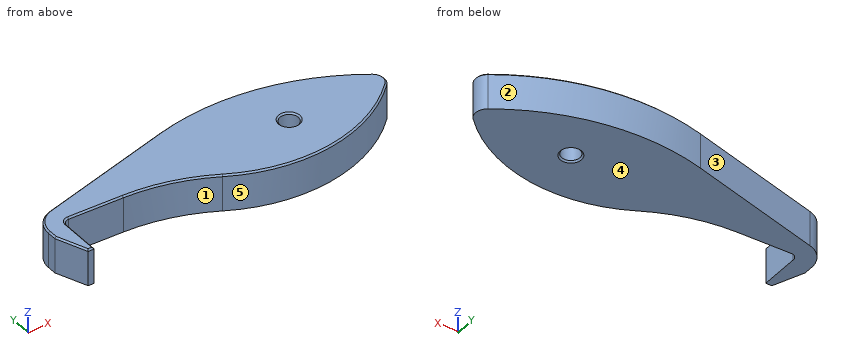
Autodesk Inventor part; units mm, degrees
ref_plane "YZ Plane" through (0, 0, 0) normal (1, 0, 0) x (0, 1, 0)
ref_plane "XZ Plane" through (0, 0, 0) normal (0, 1, 0) x (-1, 0, 0)
ref_plane "XY Plane" through (0, 0, 0) normal (0, 0, 1) x (1, 0, 0)
sketch "Náčrt1" plane through (0, 0, 0) normal (0, 0, 1) x (1, 0, 0)
  line L0 (-106.433, 0) -> (55.3696, 0)
  line L1 (0, -81.7425) -> (0, 52.651)
  circle A0 centre (0, 0) radius 3
  arc A1 (30.8349, -1.8219) -> (30.2938, 4.277) centre (28, 1) ccw
  arc A2 (-76.0338, 3.7372) -> (-82, -4) centre (-74, -4) ccw
  arc A3 (-73.9347, -2.0011) -> (-75.9978, -4.0942) centre (-74, -4) ccw
  line L2 (-75.9978, -3.9058) -> (-75.9978, -16.9058)
  line L3 (-75.9978, -16.9058) -> (-77.9978, -16.9058)
  line L4 (-77.9978, -16.9058) -> (-82, -7)
  line L5 (-82, -4) -> (-82, -7)
  arc A4 (30.2938, 4.277) -> (-31.7818, 15.3695) centre (-12.7146, -57.1663) ccw
  arc A5 (-29.0159, -10.1823) -> (30.8349, -1.8219) centre (-4.6017, 33.4519) ccw
  arc A6 (-29.0159, -10.1823) -> (-56.3536, -2.5755) centre (-58.3128, -62.5435) ccw
  line L6 (-76.0338, 3.7372) -> (-31.7818, 15.3695)
  line L7 (-73.9347, -2.0011) -> (-56.3536, -2.5755)
  dimension "d0" = 6
  dimension "d1" = 8
  dimension "d2" = 28
  dimension "d3" = 1
  dimension "d4" = 16
  dimension "d5" = 4
  dimension "d6" = 4
  dimension "d7" = 74
  dimension "d8" = 13
  dimension "d9" = 158
  dimension "d10" = 2
  dimension "d11" = 3
  dimension "d12" = 75
  dimension "d13" = 50
  dimension "d14" = 60
extrude "Vysunutí1" add sketch "Náčrt1" along normal blind 12 contours A2 L6 A4 L1 A0 L0 | L0 A0 L1 A5 A6 L7 A3 L2 L3 L4 L5 A2 | L1 A4 A1 L0 A0 | A0 L0 A1 A5 L1
chamfer "Zkosení1" distance 0.5 angle 45 15 edges at (-79.9989, -11.9529, 12) (-76.9978, -16.9058, 12) (-75.9978, -10.5, 12) (-76, -4, 12) (-75.3567, -2.5305, 12) (-65.1442, -2.2883, 12) (-42.2286, -4.7395, 12) (2.3155, -16.0673, 12) (31.9843, 1.3535, 12) (0.4784, 16.6642, 12) (-53.9078, 9.5533, 12) (-80.3352, 0.8851, 12) (-82, -5.5, 12) (-3, 0, 12) (-3, 0, 0)
properties part number "Součást22"
Here's how the part is built. I have some questions about the finished solid (model axes, mm). Face numbers are marked on the shaded views. A direction names the side the tool comes from. Give positions to 0.01 mm unless a question says otherwise; leave off trailing zeros. Order: outer loops, then holes, each group sorted by start corner. A loop starts at its lowest first (then second) coordinate and runs counter-clockwise, first axis right, second up. Notation, with made-up numbers: M -9.75,-34.75 L 30.25,-34.75 A33 cw 30.25,-0.75 Z; hole C -3.75,3 d7. An arc over 180 degrees is marked long. Use a Markdown table: item, result. Add a question column.
1. If we mould it in two halves opening along X, with no side actions, what happens to the marked faces 3, 4 and 5? For each: +X half, -X half, draft (parallel to the pull), parting line (faces both ways), or undercut.
2. I need wall thicknesses on probe 1 along X at (y, z) = (-10, 0.5); probe 2 along X at (y, z) = (-9.5, 7.5); probe 3 along Y at (x, z) = (-14, 3.25). Which ranges of each line are inside material? Lowest first, please. Write a range as from..to.
3. On a 3-axis mill with a long thin cutter (end or side, diameter ignored), from which of +Z, -Z, +X, -X, +Y, -Y can I reach the whole of each face in a straight line? I mean the marked faces 1 and 2. Say none if no direction works.
4. Suppose I cut it at C-C (x = -72.5). List the corners of the cut face in (y, z) for me.
5. Suppose I cut it at B-B (x = -60). List the corners of the cut face in (y, z) for me.
6. For pin 1 Ø6 at (x, z) = (7.5, 5) entering from -Y; pin 2 Ø4 at (x, z) = (-69, 2) entering from -Y; pin 3 Ø6 at (x, z) = (-47.5, 5.5) entering from +Y, each with a flat end and sliding along its axis, tell me the tip position at first contact or that it passes through.
7. Suppose I cut it at A-A (z = 5). List the corners of the cut face in (x, y) for me.
Results list:
| question | item | result |
|---|---|---|
| 1 | face 3 | -X half |
| 1 | face 4 | draft |
| 1 | face 5 | undercut |
| 2 | probe 1 | x = -80.79..-76, -29.34..20.14 |
| 2 | probe 2 | x = -80.99..-76, -30.27..20.99 |
| 2 | probe 3 | y = -15.66..17.82 |
| 3 | face 1 | +Z, -Z, -Y |
| 3 | face 2 | +Z, -Z, +Y |
| 4 | outline | M -2.05,0 L 4.67,0 L 4.67,11.5 L 4.15,12 L -1.55,12 L -2.05,11.5 Z |
| 5 | outline | M -2.46,0 L 7.95,0 L 7.95,11.5 L 7.43,12 L -1.96,12 L -2.46,11.5 Z |
| 6 | pin 1 | stops at y = -15.71 |
| 6 | pin 2 | stops at y = -2.23 |
| 6 | pin 3 | stops at y = 12.03 |
| 7 | outline | M -82,-7 L -78,-16.91 L -76,-16.91 L -76,-4.09 A2 cw -73.93,-2 L -56.35,-2.58 A60 cw -29.02,-10.18 A50 ccw 30.83,-1.82 A4 ccw 30.29,4.28 A75 ccw -31.78,15.37 L -76.03,3.74 A8 ccw -82,-4 Z; hole C 0,0 d6 |
